from build123d import *

# Parameters (mm, degrees)
SKETCH1_W                = 35
SKETCH1_H                = 35
SKETCH1_W_2              = 30
SKETCH1_H_2              = 30
BOSS_EXTRUDE1_DEPTH      = 45
SKETCH5_W                = 20
SKETCH5_H                = 20
BOSS_EXTRUDE3_DEPTH      = 302.5
BOSS_EXTRUDE3_DEPTH_BACK = 362.5


with BuildPart() as part:
    # Sketch1 → Boss-Extrude1 (new body)
    with BuildSketch(Plane(origin=(0, 0, 0), x_dir=(1, 0, 0), z_dir=(0, 1, 0))):
        Rectangle(SKETCH1_W, SKETCH1_H)
        Rectangle(SKETCH1_W_2, SKETCH1_H_2, mode=Mode.SUBTRACT)
    extrude(amount=-BOSS_EXTRUDE1_DEPTH)

    # Sketch5 → Boss-Extrude3 (add, two sides)
    with BuildSketch(Plane(origin=(0, 4.694715628, 18.829475929), x_dir=(1, 0, 0), z_dir=(0, -0.241921896, -0.970295726))) as boss_extrude3_sk:
        with Locations((0.25, 13.628828434)):
            Rectangle(SKETCH5_W, SKETCH5_H)
    extrude(amount=BOSS_EXTRUDE3_DEPTH)
    extrude(boss_extrude3_sk.sketch, amount=-BOSS_EXTRUDE3_DEPTH_BACK)


solid = part.part
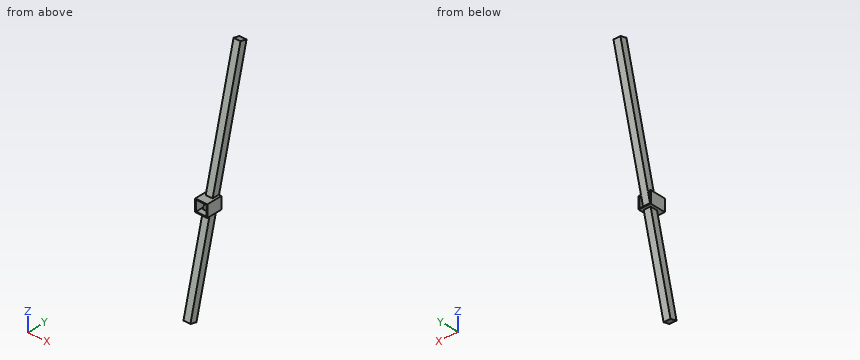
Input: part model. Units: mm. Frame: model coordinates. Give positions to 0.01 mm unless a question says otherwise; leave off trailing zeros. Loops run counter-clockwise (first coordinate to the right, second up) from the corner with the lowest first, then second, coordinate; pieces in that order, holes last. Notation, with made-up numbers: (11.25, -29.75) - (58.25, -29.75) arc R16 ccw to (58.25, -4.75) - close; hole circle Ø7 at (44, 74.5). An arc over 180 degrees is marked (long way). Use CSV: the item, a comma, the result in double quotes. Start each with the question number.
Item 1: Section D-D on z = 90.5. Return loops of the section in (x, y).
Item 2: Line query: line 1 (X direction, y = 0.5, z = 84); line 2 (Y direction, x = -8.5, z = 243.5); line 3 (Y direction, x = 5, z = 326.5). Output: solid intervals per line, ascending.
Item 3: Contact query for flat-ended pins moving along their axis: P1, Ø4, axis at x = -4, z = -22, coming from the -Y side; P2, Ø3, axis at x = -2, z = 84.5, coming from the -Y side; P3, Ø5, axis at x = 3, z = 31.5, coming from the -Y side. Output: stop coordinate, or through.
Item 4: Section C-C on y = 55. Return loops of the section in (x, z), then the cut area to 3 significant figures.
Item 5: Section A-A on y = -36. Return loops of the section in (x, z).
Item 6: Section B-B on x = 5. Return loops of the section in (y, z).
Ans:
1,outline,"(-9.75, -1.79) - (10.25, -1.79) - (10.25, 18.82) - (-9.75, 18.82) - close"
2,line 1,"x = -9.75 to 10.25"
2,line 2,"y = 36.36 to 56.97"
2,line 3,"y = 57.05 to 77.67"
3,P1,"stops at y = -30.34"
3,P2,"stops at y = -3.66"
3,P3,"stops at y = -17.12"
4,outline,"(-9.75, 235.59) - (10.25, 235.59) - (10.25, 318.26) - (-9.75, 318.26) - close"
4,area,"1,650 mm2"
5,outline,"(-17.5, -17.5) - (17.5, -17.5) - (17.5, 17.5) - (-17.5, 17.5) - close; (-9.75, -129.39) - (10.25, -129.39) - (10.25, -46.72) - (-9.75, -46.72) - close; hole (-15, -15) - (15, -15) - (15, 15) - (-15, 15) - close"
6,outline,"(-91.41, -268.97) - (-72.01, -273.81) - (-8.1, -17.5) - (0, -17.5) - (0, -15) - (-7.48, -15) - (88.87, 371.44) - (69.46, 376.28) - (-19.99, 17.5) - (-45, 17.5) - (-45, 15) - (-20.61, 15) - (-28.09, -15) - (-45, -15) - (-45, -17.5) - (-28.72, -17.5) - close"
